Input: part model. Units: mm. Frame: model coordinates. A direction names the side the tool comes from. Coordinates: 2 decimals unless noted, no trailing zeros. Order: outer loops, then holes, each group sorted by start corner. A loop starts at its lowest first (then second) coordinate and runs counter-clockwise, first axis right, second up.
from build123d import *

# Parameters (mm, degrees)
BOSS_EXTRUDE1_DEPTH      = 500
BOSS_EXTRUDE1_DEPTH_BACK = 500


with BuildPart() as part:
    # Sketch1 → Boss-Extrude1 (new body, two sides)
    with BuildSketch(Plane.XY) as boss_extrude1_sk:
        with BuildLine():
            Line((-14, -16), (14, -16))
            ThreePointArc((14, -16), (15.414213562, -15.414213562), (16, -14))
            Line((16, -14), (16, 14))
            ThreePointArc((16, 14), (15.414213562, 15.414213562), (14, 16))
            Line((14, 16), (-14, 16))
            ThreePointArc((-14, 16), (-15.414213562, 15.414213562), (-16, 14))
            Line((-16, 14), (-16, -14))
            ThreePointArc((-16, -14), (-15.414213562, -15.414213562), (-14, -16))
        make_face()
        with BuildLine():
            Line((-14, 14.48), (14, 14.48))
            ThreePointArc((14, 14.48), (14.339411255, 14.339411255), (14.48, 14))
            Line((14.48, 14), (14.48, -14))
            ThreePointArc((14.48, -14), (14.339411255, -14.339411255), (14, -14.48))
            Line((14, -14.48), (-14, -14.48))
            ThreePointArc((-14, -14.48), (-14.339411255, -14.339411255), (-14.48, -14))
            Line((-14.48, -14), (-14.48, 14))
            ThreePointArc((-14.48, 14), (-14.339411255, 14.339411255), (-14, 14.48))
        make_face(mode=Mode.SUBTRACT)
    extrude(amount=BOSS_EXTRUDE1_DEPTH)
    extrude(boss_extrude1_sk.sketch, amount=-BOSS_EXTRUDE1_DEPTH_BACK)


solid = part.part
Item 1: Pin query (flat end, axial travel): pin 1 Ø10 at (x, y) = (10, 0) entering from -Z. Return the tip coordinate at first contact, or that it passes through.
Response values:
pin 1: stops at z = -500
Item 2: Access query for faces 1 (the face through (0, 16, 7)), 2 (the face through (0, -14.48, 7)). Directions: +Z, -Z, +X, -X, +Y, -Y. A direction counts if a zero-diameter tool reaches every point of the face in a straight line with its end or side. Return the directions, or none.
Response values:
face 1: +Z, -Z, +X, -X, +Y
face 2: +Z, -Z
Item 3: Cut plane C-C on z = 323.5. Return loops of the section in (x, y), then the cut area to 3 significant figures.
Response values:
outline: (-16, -14) arc R2 ccw to (-14, -16) - (14, -16) arc R2 ccw to (16, -14) - (16, 14) arc R2 ccw to (14, 16) - (-14, 16) arc R2 ccw to (-16, 14) - close; hole (-14.48, -14) arc R0.48 ccw to (-14, -14.48) - (14, -14.48) arc R0.48 ccw to (14.48, -14) - (14.48, 14) arc R0.48 ccw to (14, 14.48) - (-14, 14.48) arc R0.48 ccw to (-14.48, 14) - close
area: 182 mm2
Item 4: Cut plane A-A on x = -9. Return loops of the section in (y, z).
Response values:
outline: (-16, -500) - (-14.48, -500) - (-14.48, 500) - (-16, 500) - close; (14.48, -500) - (16, -500) - (16, 500) - (14.48, 500) - close
Item 5: Ray query, probe 1 along Y at (x, z) = (12, 459.5); probe 2 along X at (y, z) = (-15, 460.5). Return the intervals inside material, ascending.
Response values:
probe 1: y = -16 to -14.48, 14.48 to 16
probe 2: x = -15.73 to 15.73
